Input: dimensioned drawing with shaded views. Units: mm. Origin: part minimum x, y, z. Give positions to 0.01 mm unless a question says otherwise; leave off trailing zeros. Order: outer loops, then holes, each group sorted by start corner. A loop starts at its lowest first (then second) coordinate and runs counter-clockwise, first axis right, second up. Notation, with made-up numbers: (-15.75, 32.5) - (42.25, 32.5) arc R20 ccw to (42.25, 62.5) - close; hole circle Ø6 at (78, 25.5). An arc over 180 degrees is marked (long way). Use a Markdown table: item, result.
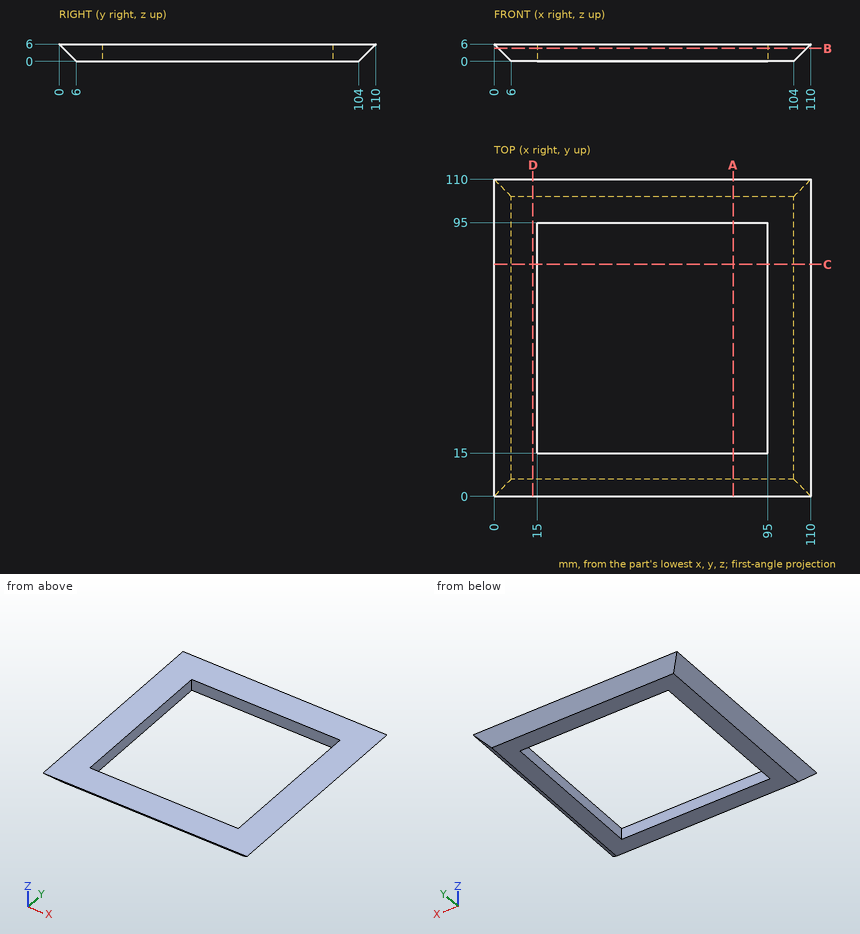
1. Section query D-D (x = 13.5). Return loops of the section in (y, z).
Response:
| item | result |
|---|---|
| outline | (0, 6) - (6, 0) - (104, 0) - (110, 6) - close |
2. Section query A-A (x = 83). Return loops of the section in (y, z), then the cut area to 3 significant figures.
Response:
| item | result |
|---|---|
| outline | (0, 6) - (6, 0) - (15, 0) - (15, 6) - close; (95, 0) - (104, 0) - (110, 6) - (95, 6) - close |
| area | 144 mm^2 |
3. Section query B-B (z = 4.5). Return loops of the section in (x, y).
Response:
| item | result |
|---|---|
| outline | (1.5, 1.5) - (108.5, 1.5) - (108.5, 108.5) - (1.5, 108.5) - close; hole (15, 15) - (95, 15) - (95, 95) - (15, 95) - close |
4. Pin query (flat end, axial travel): pin 1 (1 mm diameter, centred on y = 19, z = 4.5, fed in from -X); pin 2 (3 mm diameter, centred on y = 62, z = 1.5, fed in from +X); pin 3 (3 mm diameter, centred on x = 71, z = 2, fed in from -Y). Return the tip coordinate at first contact, or that it passes through.
Response:
| item | result |
|---|---|
| pin 1 | stops at x = 1 |
| pin 2 | stops at x = 107 |
| pin 3 | stops at y = 2.5 |
5. Material intervals for line 1 along Y through (x, z) = (51.5, 1); line 2 along X through (y, z) = (58.5, 5.5); line 3 along X through (y, z) = (56, 2.5), sorted ascending.
Response:
| item | result |
|---|---|
| line 1 | y = 5 to 15, 95 to 105 |
| line 2 | x = 0.5 to 15, 95 to 109.5 |
| line 3 | x = 3.5 to 15, 95 to 106.5 |
